```python
from build123d import *

# Parameters (mm, degrees)
BOSS_EXTRUDE1_DEPTH       = 64
SKETCH2_W                 = 100
SKETCH2_H                 = 50
BOSS_EXTRUDE2_DEPTH       = 4
BOSS_EXTRUDE3_DEPTH       = 4
SKETCH4_W                 = 25
SKETCH4_H                 = 35
BOSS_EXTRUDE4_DEPTH       = 4
F_6_0MM_START             = -4
F_6_0MM_DOWEL_SLOT1_DEPTH = 4
CHAMFER1_SIZE             = 10
CHAMFER2_SIZE             = 2
FILLET1_R                 = 3


# Read off the part's stored shape, not the designer's step: Ø6.0mm Dowel Slot1
with BuildPart() as part:
    # Sketch1 → Boss-Extrude1 (new body)
    with BuildSketch(Plane(origin=(0, 0, 0), x_dir=(1, 0, 0), z_dir=(0, 1, 0))):
        Polygon((0, 0), (0, 4), (-100, 4), (-100, -46), (-96, -46), (-96, 0), align=None)
    extrude(amount=BOSS_EXTRUDE1_DEPTH)

    # Sketch2 → Boss-Extrude2 (add)
    with BuildSketch(Plane.XZ):
        with Locations((-50, 21)):
            Rectangle(SKETCH2_W, SKETCH2_H)
    extrude(amount=BOSS_EXTRUDE2_DEPTH)

    # Sketch3 → Boss-Extrude3 (add)
    with BuildSketch(Plane(origin=(0, 64, 0), x_dir=(1, 0, 0), z_dir=(0, 1, 0))):
        Polygon((-96, 0), (-81, 0), (-96, -15), align=None)
    extrude(amount=-BOSS_EXTRUDE3_DEPTH)

    # Sketch4 → Boss-Extrude4 (add)
    with BuildSketch(Plane.XZ.offset(4)):
        with Locations((-40, -21.5)):
            Rectangle(SKETCH4_W, SKETCH4_H)
    extrude(amount=-BOSS_EXTRUDE4_DEPTH)

    # Ø6.0mm Dowel Slot1 outline → Ø6.0mm Dowel Slot1 (cut)
    with BuildSketch(Plane(origin=(0, 0, 0), x_dir=(1, 0, 0), z_dir=(0, 1, 0)).offset(F_6_0MM_START)):
        with BuildLine():
            Line((-45.25, 10.75), (-34.75, 10.75))
            ThreePointArc((-34.75, 10.75), (-31.5, 14), (-34.75, 17.25))
            Line((-34.75, 17.25), (-45.25, 17.25))
            ThreePointArc((-45.25, 17.25), (-48.5, 14), (-45.25, 10.75))
        make_face()
        with BuildLine():
            Line((-45.25, 25.75), (-34.75, 25.75))
            ThreePointArc((-34.75, 25.75), (-31.5, 29), (-34.75, 32.25))
            Line((-34.75, 32.25), (-45.25, 32.25))
            ThreePointArc((-45.25, 32.25), (-48.5, 29), (-45.25, 25.75))
        make_face()
    extrude(amount=F_6_0MM_DOWEL_SLOT1_DEPTH, mode=Mode.SUBTRACT)

    # Chamfer1
    chamfer1_edges = [part.edges().sort_by_distance(p)[0] for p in [
        (-52.5, -2, -4),
        (-27.5, -2, -4),
    ]]
    chamfer(chamfer1_edges, length=CHAMFER1_SIZE)

    # Chamfer2
    chamfer2_edges = [part.edges().sort_by_distance(p)[0] for p in [
        (-52.5, -2, -39),
        (-27.5, -2, -39),
    ]]
    chamfer(chamfer2_edges, length=CHAMFER2_SIZE)

    # Fillet1
    fillet1_edges = [part.edges().sort_by_distance(p)[0] for p in [
        (-40, 0, -4),
    ]]
    fillet(fillet1_edges, radius=FILLET1_R)


solid = part.part
```
Geometry check sheet. Reference: the model listing, model coordinates, mm. A direction names the side the tool comes from. Round coordinates to 2 decimals unless told otherwise and drop trailing zeros. Loops run counter-clockwise (first coordinate to the right, second up) from the corner with the lowest first, then second, coordinate; pieces in that order, holes last. Notation, with made-up numbers: (75, 34) - (109, 34) arc R20 cw to (109, 67) - close; hole circle Ø10 at (-28.5, 4.5). An arc over 180 degrees is marked (long way). Write each question's results on one line, items separated by ' | '. Start each with the question number.
Q1. Cross-section at C-C on y = 52.5. Enter the section's corners in (x, z), and give its area (3 significant figures).
Q2. Gauge pin test, flat ends, axial feed: P1, Ø3, axis at y = -2.5, z = -29, coming from the +X side; P2, Ø3, axis at x = -51, z = 21, coming from the +Y side; P3, Ø4, axis at x = -82.5, y = 52.5, coming from the +Z side. Record the tip position at first contact, or that the pin passes through.
Q3. Cross-section at A-A on x = -93. Enter the section's corners in (y, z).
Q4. Cross-section at B-B on z = -29. Enter the section's corners in (x, y), and give its area (3 significant figures).
Q5. Release check for a two-part mould opening along Y. For faces 1 (the flat face through (-92, 60, 4)), 2 (the flat face through (-40, -2, -25.75)), 3 (the cylindrical face through (-40.32, 0.86, -4.9)) record: +Y half, -Y half, draft (parallel to the pull), parting line (faces both ways), or undercut.
Q6. Thickness scan on line 1 (Z direction, x = -59.5, y = 53.5); line 2 (X direction, y = 6.5, z = 19). Record the ranges inside material, lowest first. Write a range as [from, to].
Q7. Access from +Z, -Z, +X, -X, +Y, -Y to the whole of each face (thin tool, end or side, straight path). Record for faces 4 (the flat face through (-40, -2, -39)), 5 (the flat face through (-65, -3, 46)), 6 (the flat face through (-88, 62, 7)), 7 (the flat face through (-40, -2, -32.25)), 8 (the flat face through (-52.5, -2, -26)).
Q8. Cross-section at D-D on z = 35.5. Enter the section's corners in (x, y), and give its area (3 significant figures).
Answers below:
1) outline: (-100, -4) - (0, -4) - (0, 0) - (-96, 0) - (-96, 46) - (-100, 46) - close | area: 584 mm²
2) P1: stops at x = -27.5 | P2: stops at y = 0 | P3: stops at z = 0
3) outline: (-4, -4) - (64, -4) - (64, 12) - (60, 12) - (60, 0) - (0, 0) - (0, 46) - (-4, 46) - close
4) outline: (-52.5, -4) - (-48.5, -4) - (-48.5, 0) - (-52.5, 0) - close; (-31.5, -4) - (-27.5, -4) - (-27.5, 0) - (-31.5, 0) - close | area: 32.0 mm²
5) face 1: undercut | face 2: draft | face 3: +Y half
6) line 1: z = [-4, 0] | line 2: x = [-100, -96]
7) face 4: -Z, +X, -X, +Y, -Y | face 5: +Z, +X, -X, +Y, -Y | face 6: +Z, +X, +Y | face 7: +Y, -Y | face 8: -Z, -X, +Y, -Y
8) outline: (-100, -4) - (0, -4) - (0, 0) - (-96, 0) - (-96, 64) - (-100, 64) - close | area: 656 mm²
